```python
from build123d import *

# Parameters (mm, degrees)
BOSS_EXTRUDE1_DEPTH     = 5
F_8_0MM_DOWEL_HOLE1_D   = 8
BOSS_EXTRUDE2_DEPTH     = 10
CUT_EXTRUDE1_DEPTH      = 136.922772191
CUT_EXTRUDE1_DEPTH_BACK = 136.922772191


with BuildPart() as part:
    # Sketch1 → Boss-Extrude1 (new, symmetric)
    with BuildSketch(Plane.XY):
        with BuildLine():
            Line((-125, 10), (125, 10))
            ThreePointArc((125, 10), (135, 0), (125, -10))
            Line((125, -10), (-125, -10))
            ThreePointArc((-125, -10), (-135, 0), (-125, 10))
        make_face()
    extrude(amount=BOSS_EXTRUDE1_DEPTH, both=True)

    # Ø8.0mm Dowel Hole1 (through all)
    with Locations(Plane.XY.offset(5)):
        with Locations((-125, 0), (125, 0)):
            Hole(F_8_0MM_DOWEL_HOLE1_D / 2)

    # Sketch4 → Boss-Extrude2 (add)
    with BuildSketch(Plane.XY.offset(5)):
        with BuildLine():
            Line((-5, 10), (5, 10))
            ThreePointArc((5, 10), (1.464466094, 11.464466094), (0, 15))
            ThreePointArc((0, 15), (-1.464466094, 11.464466094), (-5, 10))
        make_face()
    extrude(amount=-BOSS_EXTRUDE2_DEPTH)

    # Sketch5 → Cut-Extrude1 (cut, two sides: drawn at the far end of the back side and taken through both)
    with BuildSketch(Plane(origin=(0, 0, 0), x_dir=(0, 0, -1), z_dir=(1, 0, 0)).offset(-CUT_EXTRUDE1_DEPTH_BACK)):
        with BuildLine():
            Line((-5, 10), (-5, 20))
            Line((-5, 20), (5, 20))
            Line((5, 20), (5, 10))
            ThreePointArc((5, 10), (1.464466094, 11.464466094), (0, 15))
            ThreePointArc((0, 15), (-1.464466094, 11.464466094), (-5, 10))
        make_face()
    extrude(amount=CUT_EXTRUDE1_DEPTH + CUT_EXTRUDE1_DEPTH_BACK, mode=Mode.SUBTRACT)


solid = part.part
```
The listing builds one solid part. Answer for the finished solid, in the listing's coordinates (mm). A direction names the side the tool comes from. Give positions to 0.01 mm unless a question says otherwise; leave off trailing zeros. Loops run counter-clockwise (first coordinate to the right, second up) from the corner with the lowest first, then second, coordinate; pieces in that order, holes last. Notation, with made-up numbers: (15, 65) - (29, 65) arc R19 cw to (29, 76) - close; hole circle Ø9 at (12.25, 56.25). An arc over 180 degrees is marked (long way). Return JSON: item names as keys, results as strings. Group by question number.
1. Find section D-D (x = 76). Write down the section's boundary in (y, z), then the cut area to 3 significant figures.
2. Find section A-A (y = 0). Write down the section's boundary in (x, z).
3. Given pin 1 Ø6 at (x, z) = (42.5, -3) entering from +Y, flat-ended and moving along its own axis, determine where the tip first touches the part or whether it passes through.
4. Find section C-C (x = -2.5). Write down the section's boundary in (y, z), then the cut area to 3 significant figures.
5. Find section B-B (z = -2). Write down the section's boundary in (x, y).
6. Straight lines are drawn through the part: line 1 (Y direction, x = -125, z = -0.25); line 2 (X direction, y = 3.5, z = -2); line 3 (X direction, y = 1.25, z = -0.75). For each, find the intervals that lie inside material, in ascending order. Write a range as [from, to].
7. Which of the six approach directions +Z, -Z, +X, -X, +Y, -Y give full straight-line access (tool end or side, diameter ignored) to faces 5 (the cylindrical face through (-0.07, 10.446, -2.937)), 6 (the flat face through (-66, 10, 0))?
8. Determine the mould class of faces 1 (the cylindrical face through (-135, 0, 0)), 2 (the cylindrical face through (-121, 0, 0)), 3 (the flat face through (64, 10, 0)), 4 (the cylindrical face through (121.305, -1.532, -0.07)) for opening direction X: pulls with the +X half, pulls with the -X half, needs draft (parallel to the pull), parting line crosses it, or undercut.
Verdict:
{
 "1": {"outline": "(-10, -5) - (10, -5) - (10, 5) - (-10, 5) - close", "area": "200 mm^2"},
 "2": {"outline": "(-135, -5) - (-129, -5) - (-129, 5) - (-135, 5) - close; (-121, -5) - (121, -5) - (121, 5) - (-121, 5) - close; (129, -5) - (135, -5) - (135, 5) - (129, 5) - close"},
 "3": {"pin 1": "stops at y = 10"},
 "4": {"outline": "(-10, -5) - (10, -5) arc R5 cw to (10.67, -2.5) - (10.67, 2.5) arc R5 cw to (10, 5) - (-10, 5) - close", "area": "204 mm^2"},
 "5": {"outline": "(-125, -10) - (125, -10) arc R10 ccw to (125, 10) - (5, 10) arc R5 cw to (2, 11) - (-2, 11) arc R5 cw to (-5, 10) - (-125, 10) arc R10 ccw to start; hole circle Ø8 at (-125, 0); hole circle Ø8 at (125, 0)"},
 "6": {"line 1": "y = [-10, -4], [4, 10]", "line 2": "x = [-134.37, -126.94], [-123.06, 123.06], [126.94, 134.37]", "line 3": "x = [-134.92, -128.8], [-121.2, 121.2], [128.8, 134.92]"},
 "7": {"face 5": "-Z, +X, -X, +Y", "face 6": "+Z, -Z, -X, +Y"},
 "8": {"face 1": "pulls with the -X half", "face 2": "undercut", "face 3": "needs draft", "face 4": "undercut"}
}
